from build123d import *

# Parameters (mm, degrees)
F0_W     = 36.20262
F0_H     = 1.89738
F1_DEPTH = 304.8
F2_R     = 7.14375
F3_DEPTH = 25.4
F4_R     = 7.14375
F5_DEPTH = 25.4


with BuildPart() as f1:
    # F0 (on Front) → F1 (new body)
    with BuildSketch(Plane.XZ):
        with Locations((19.99869, 0.94869)):
            Rectangle(F0_W, F0_H)
        Polygon((0, 38.1), (0, 0), (1.89738, 0), (1.89738, 1.89738), (1.89738, 38.1), align=None)
    extrude(amount=F1_DEPTH)

    # F2 (on face) → F3 (cut)
    with BuildSketch(Plane.XY.offset(1.89738)):
        with Locations((19.05, -271.4625)):
            Circle(F2_R)
        with Locations((19.05, -223.8375)):
            Circle(F2_R)
        with Locations((19.05, -176.2125)):
            Circle(F2_R)
        with Locations((19.05, -128.5875)):
            Circle(F2_R)
        with Locations((19.05, -80.9625)):
            Circle(F2_R)
        with Locations((19.05, -33.3375)):
            Circle(F2_R)
    extrude(amount=-F3_DEPTH, mode=Mode.SUBTRACT)

    # F4 (on face) → F5 (cut)
    with BuildSketch(Plane.YZ.offset(1.89738)):
        with Locations((-271.4625, 19.05)):
            Circle(F4_R)
        with Locations((-223.8375, 19.05)):
            Circle(F4_R)
        with Locations((-176.2125, 19.05)):
            Circle(F4_R)
        with Locations((-128.5875, 19.05)):
            Circle(F4_R)
        with Locations((-80.9625, 19.05)):
            Circle(F4_R)
        with Locations((-33.3375, 19.05)):
            Circle(F4_R)
    extrude(amount=-F5_DEPTH, mode=Mode.SUBTRACT)


solid = f1.part
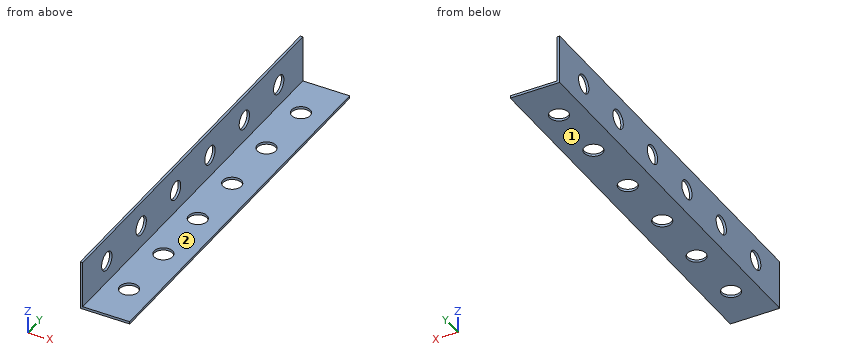
Design review of the part built by this model. Coordinates are the model's own, in mm. Face numbers are marked on the shaded views. A direction names the side the tool comes from. Give positions to 0.01 mm unless a question says otherwise; leave off trailing zeros. Loops run counter-clockwise (first coordinate to the right, second up) from the corner with the lowest first, then second, coordinate; pieces in that order, holes last. Notation, with made-up numbers: (-37.5, -37.75) -> (15.5, -37.75) arc R14 ccw to (15.5, -20.75) -> close; hole circle Ø5 at (83.5, -15). An arc over 180 degrees is marked (long way). One line per question, with ' | ' between items. Start each with the question number.
(1) For the marked faces 1 and 2, list the 3-axis set-ups (+Z, -Z, +X, -X, +Y, -Y) from which the entire face can be reached by the end or side of a thin tool; tool diameter is ignored.
(2) We need section D-D (y = -165). State the section outline as (x, z) points, and give its area (3 significant figures).
(3) We need section A-A (z = 19.05). State the section outline as (x, y) points.
(4) For line 1 (X direction, y = -231.5, z = 7.5), list the stretches that pass through material, from the lowest coordinate up.
(5) We need section B-B (x = 19.05). State the section outline as (y, z) points, and give its area (3 significant figures).
(6) Insertion check: P1, Ø13, axis at y = -176.21, z = 19.05, coming from the +X side; P2, Ø16.5, axis at x = 19.05, y = -128.59, coming from the +Z side; P3, Ø11, axis at y = -178.5, z = 24, coming from the +X side. Each pin has a flat end and moves straight along its axis. Give the tip position at first contact, or say it passes through.
(7) We need section C-C (y = -37.5). State the section outline as (x, z) points.
The answers:
1) face 1: -Z, +X, -X, +Y, -Y | face 2: +Z, +X, +Y, -Y
2) outline: (0, 0) -> (38.1, 0) -> (38.1, 1.9) -> (1.9, 1.9) -> (1.9, 38.1) -> (0, 38.1) -> close | area: 141 mm^2
3) outline: (0, -304.8) -> (1.9, -304.8) -> (1.9, -278.61) -> (0, -278.61) -> close; (0, -264.32) -> (1.9, -264.32) -> (1.9, -230.98) -> (0, -230.98) -> close; (0, -216.69) -> (1.9, -216.69) -> (1.9, -183.36) -> (0, -183.36) -> close; (0, -169.07) -> (1.9, -169.07) -> (1.9, -135.73) -> (0, -135.73) -> close; (0, -121.44) -> (1.9, -121.44) -> (1.9, -88.11) -> (0, -88.11) -> close; (0, -73.82) -> (1.9, -73.82) -> (1.9, -40.48) -> (0, -40.48) -> close; (0, -26.19) -> (1.9, -26.19) -> (1.9, 0) -> (0, 0) -> close
4) line 1: x = 0 to 1.9
5) outline: (-304.8, 0) -> (-278.61, 0) -> (-278.61, 1.9) -> (-304.8, 1.9) -> close; (-264.32, 0) -> (-230.98, 0) -> (-230.98, 1.9) -> (-264.32, 1.9) -> close; (-216.69, 0) -> (-183.36, 0) -> (-183.36, 1.9) -> (-216.69, 1.9) -> close; (-169.07, 0) -> (-135.73, 0) -> (-135.73, 1.9) -> (-169.07, 1.9) -> close; (-121.44, 0) -> (-88.11, 0) -> (-88.11, 1.9) -> (-121.44, 1.9) -> close; (-73.82, 0) -> (-40.48, 0) -> (-40.48, 1.9) -> (-73.82, 1.9) -> close; (-26.19, 0) -> (0, 0) -> (0, 1.9) -> (-26.19, 1.9) -> close | area: 416 mm^2
6) P1: passes through | P2: stops at z = 1.9 | P3: stops at x = 1.9
7) outline: (0, 0) -> (13.24, 0) -> (13.24, 1.9) -> (1.9, 1.9) -> (1.9, 13.24) -> (0, 13.24) -> close; (0, 24.86) -> (1.9, 24.86) -> (1.9, 38.1) -> (0, 38.1) -> close; (24.86, 0) -> (38.1, 0) -> (38.1, 1.9) -> (24.86, 1.9) -> close
